The listing builds one solid part. Answer for the finished solid, in the listing's coordinates (mm). A direction names the side the tool comes from. Coordinates: 2 decimals unless noted, no trailing zeros. Return JSON: item names as keys, results as strings.
```python
from build123d import *

# Parameters (mm, degrees)
SKETCH2_R          = 2
CUT_EXTRUDE1_DEPTH = 10
SKETCH3_R          = 2
CUT_EXTRUDE2_DEPTH = 10
CIRPATTERN1_COUNT  = 20


with BuildPart() as part:
    # Sketch1 → Revolve1 (revolve)
    with BuildSketch(Plane.XY, mode=Mode.PRIVATE) as revolve1_sk:
        with BuildLine():
            Line((125.35, 214), (125.35, 182))
            Line((125.35, 182), (90.777397171, 182))
            ThreePointArc((90.777397171, 182), (76.303023046, 182.019382519), (61.85, 181.233248409))
            Line((61.85, 181.233248409), (61.85, 176.215984101))
            ThreePointArc((61.85, 176.215984101), (50.315984949, 174.982485494), (38.85, 173.225723944))
            Line((38.85, 173.225723944), (38.85, 178.301556459))
            ThreePointArc((38.85, 178.301556459), (20.180307559, 174.359561219), (1.85, 169.058941719))
            Line((1.85, 169.058941719), (1.85, 163.789069776))
            ThreePointArc((1.85, 163.789069776), (-9.759071612, 159.566063637), (-21.15, 154.785783832))
            Line((-21.15, 154.785783832), (-21.15, 160.254972016))
            ThreePointArc((-21.15, 160.254972016), (-39.005794183, 151.605014565), (-56.15, 141.618656033))
            Line((-56.15, 141.618656033), (-56.15, 103))
            Line((-56.15, 103), (-85.15, 95))
            Line((-85.15, 95), (-125.15, 95))
            Line((-125.15, 95), (-125.15, 130))
            Line((-125.15, 130), (-120.15, 130))
            Line((-120.15, 130), (-120.15, 100))
            Line((-120.15, 100), (-85.827011196, 100))
            Line((-85.827011196, 100), (-61.15, 106.807451364))
            Line((-61.15, 106.807451364), (-61.15, 144.350032201))
            ThreePointArc((-61.15, 144.350032201), (-39.212159428, 157.147213449), (-16.15, 167.785516856))
            Line((-16.15, 167.785516856), (-16.15, 162.383703009))
            ThreePointArc((-16.15, 162.383703009), (-9.683274673, 164.95660686), (-3.15, 167.355500925))
            Line((-3.15, 167.355500925), (-3.15, 172.650142104))
            ThreePointArc((-3.15, 172.650142104), (20.086400181, 179.487164129), (43.85, 184.174006054))
            Line((43.85, 184.174006054), (43.85, 179.116880269))
            ThreePointArc((43.85, 179.116880269), (50.339565328, 180.026751253), (56.85, 180.772783246))
            Line((56.85, 180.772783246), (56.85, 185.798153237))
            ThreePointArc((56.85, 185.798153237), (73.830693152, 186.94526342), (90.85, 187))
            Line((90.85, 187), (120.35, 187))
            Line((120.35, 187), (120.35, 214))
            Line((120.35, 214), (125.35, 214))
        make_face()
    revolve(revolve1_sk.sketch.rotate(Axis((-99.349120664, 0, 0), (1, 0, 0)), 90), axis=Axis((-99.349120664, 0, 0), (1, 0, 0)))

    # Sketch2 → Cut-Extrude1 (cut)
    with BuildSketch(Plane.ZY.offset(125.15)):
        with Locations((0, 122.5)):
            Circle(SKETCH2_R)
    cut_extrude1 = extrude(amount=-CUT_EXTRUDE1_DEPTH, mode=Mode.SUBTRACT)

    # Sketch3 → Cut-Extrude2 (cut)
    with BuildSketch(Plane(origin=(125.35, 0, 0), x_dir=(0, 0, -1), z_dir=(1, 0, 0))):
        with Locations((0, 200)):
            Circle(SKETCH3_R)
    cut_extrude2 = extrude(amount=-CUT_EXTRUDE2_DEPTH, mode=Mode.SUBTRACT)

    # CirPattern1: Cut-Extrude1, Cut-Extrude2 ×20 about axis
    cirpattern1_axis = Axis((0, 0, 0), (1, 0, 0))
    add([cut_extrude1.rotate(cirpattern1_axis, i * 360 / CIRPATTERN1_COUNT) for i in range(1, CIRPATTERN1_COUNT)], mode=Mode.SUBTRACT)
    add([cut_extrude2.rotate(cirpattern1_axis, i * 360 / CIRPATTERN1_COUNT) for i in range(1, CIRPATTERN1_COUNT)], mode=Mode.SUBTRACT)


solid = part.part
```
Item 1: Which of the six approach directions +Z, -Z, +X, -X, +Y, -Y give full straight-line access (tool end or side, diameter ignored) to faces 4 (the flat face through (-16.15, -137, -88)), 5 (the flat face through (-125.15, -68, -67)), 6 (the flat face through (-56.15, 104, 10)), 7 (the cylindrical face through (-122.615, -39.048, 123.997)), 8 (the cylindrical face through (-105.43, 92.74, -20.59))?
Answer list:
{"face 4": "none", "face 5": "+Z, -Z, -X, +Y, -Y", "face 6": "+X", "face 7": "-X", "face 8": "+X, -X"}
Item 2: Find the intervals of material crossed by probe 1 along Y at (x, z) = (-91, 3.5); probe 2 along Z at (x, y) = (-5.5, 64); probe 3 along X at (y, z) = (108, -117), in increasing order.
Answer list:
{"probe 1": "-99.94 to -94.94, 94.94 to 99.94", "probe 2": "-153.73 to -147.94, 147.94 to 153.73", "probe 3": "-35.13 to -23.47, -21.15 to -10.62"}
Item 3: Determine the mould class of faces 1 (the cylindrical face through (107.822, -54.668, 173.596)), 2 (the flat face through (125.35, -144, -112)), 3 (the flat face through (-61.15, -108, 1)) for opening direction X: pulls with the +X half, pulls with the -X half, needs draft (parallel to the pull), parting line crosses it, or undercut.
Answer list:
{"face 1": "needs draft", "face 2": "pulls with the +X half", "face 3": "undercut"}
Item 4: Flat-ended cylindrical pins translate along their axes: pin 1 (3 mm diameter, centred on x = -37, z = -54, fed in from -Y); pin 2 (2.5 mm diameter, centred on y = -117.56, z = 161.8, fed in from -X); pin 3 (4 mm diameter, centred on x = 92, y = -13.5, fed in from +Z); pin 4 (6 mm diameter, centred on x = 33, z = -110.5, fed in from -Y). Find the tip coordinate at first contact, or state that the pin passes through.
Answer list:
{"pin 1": "y = -149.76", "pin 2": "through", "pin 3": "z = 186.65", "pin 4": "y = -147.36"}
